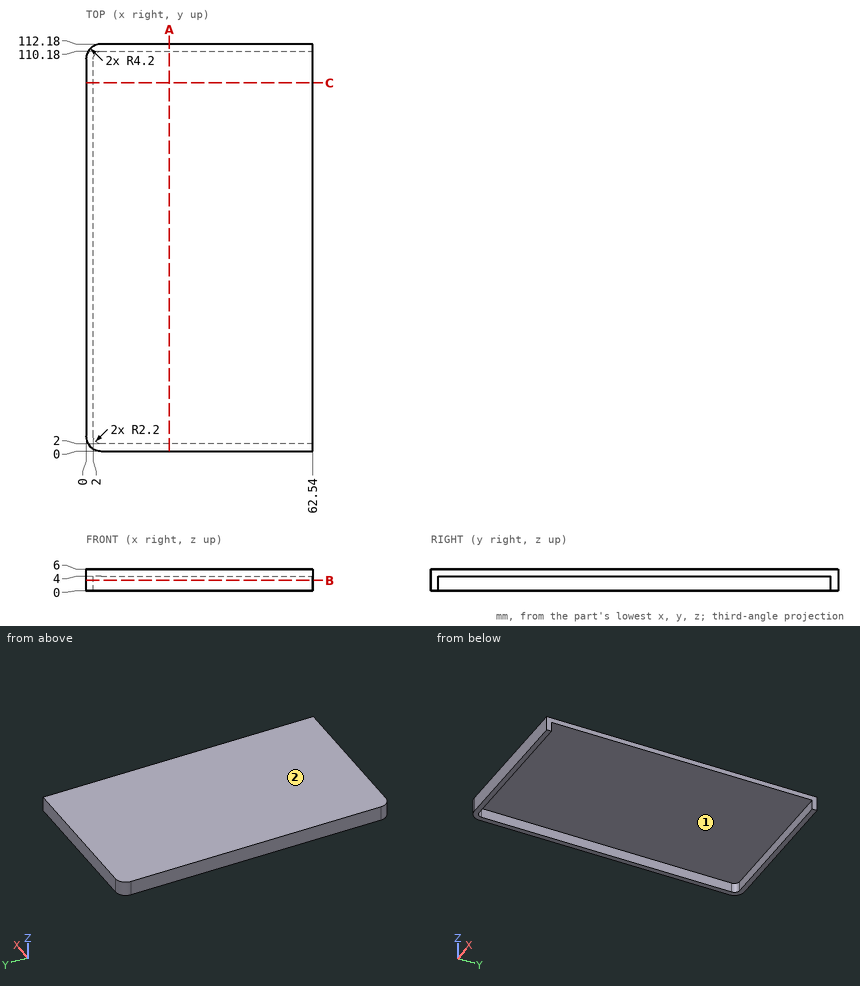
The drawing under review shows one solid part. Ordinate dimensions are in mm from its lowest x, y, z. Round coordinates to 2 decimals unless told otherwise and drop trailing zeros. Write each loop counter-clockwise with the first axis right and the second up, starting at its lowest first coordinate (ties: lowest second). Pieces come first, ordered by that corner, then holes. Notation, with made-up numbers: M -22.5,43.5 L -10.5,43.5 A9 cw -10.5,51.5 Z; hole C 24.5,87.25 d6. An arc over 180 degrees is marked long. One line per item, written item: value. Start each with the question number.
(1) The part is to be moulded in two halves that separate along Y. For the marked faces 1 and 2, say which applies: released by +Y, released by -Y, zero draft, split by the parting line, or undercut.
(2) Insertion check: pin 1 (4 mm diameter, centred on x = 18.5, y = 29, fed in from -Z); pin 2 (1.2 mm diameter, centred on y = 32.5, z = 3, fed in from +X). Each pin has a flat end and moves straight along its axis. Give the tip position at first contact, or say it passes through.
(3) Wall thickness on line 1 (Y direction, x = 30, z = 2.9); line 2 (Z direction, x = 41.5, y = 45); line 3 (X direction, y = 49, z = 1.7): over which ranges is each line inside the solid? List them lowest first.
(4) We need section B-B (z = 2.9). Give the boundary of the cut face in (x, y).
(5) We need section C-C (y = 101.5). Give the boundary of the cut face in (x, z), and give its area (3 significant figures).
(6) We need section A-A (x = 23). Give the boundary of the cut face in (y, z).
Result:
1. face 1: undercut
1. face 2: zero draft
2. pin 1: z = 4
2. pin 2: x = 2
3. line 1: 0 to 2, 110.18 to 112.18
3. line 2: 4 to 6
3. line 3: 0 to 2
4. outline: M 0,4.2 A4.2 ccw 4.2,0 L 62.54,0 L 62.54,2 L 4.2,2 A2.2 cw 2,4.2 L 2,107.98 A2.2 cw 4.2,110.18 L 62.54,110.18 L 62.54,112.18 L 4.2,112.18 A4.2 ccw 0,107.98 Z
5. outline: M 0,0 L 2,0 L 2,4 L 62.54,4 L 62.54,6 L 0,6 Z
5. area: 133 mm²
6. outline: M 0,0 L 2,0 L 2,4 L 110.18,4 L 110.18,0 L 112.18,0 L 112.18,6 L 0,6 Z
